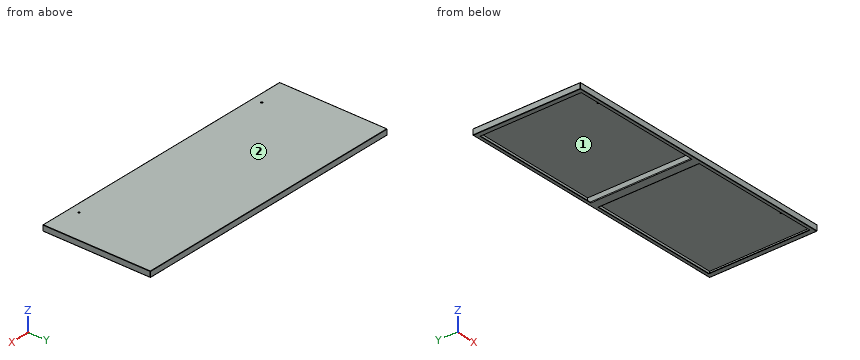
```python
from build123d import *

# Parameters (mm, degrees)
SKETCH_1_W          = 878
SKETCH_1_H          = 338
EXTRUDE_1_DEPTH     = 1.5
SKETCH_2_W          = 878
SKETCH_2_H          = 338
SKETCH_2_W_2        = 875
SKETCH_2_H_2        = 335
EXTRUDE_2_DEPTH     = 15
SKETCH_3_W          = 878
SKETCH_3_H          = 338
SKETCH_3_W_2        = 848
SKETCH_3_H_2        = 318
EXTRUDE_3_DEPTH     = 1.5
SKETCH_6_R          = 3
CUT_EXTRUDE_1_DEPTH = 471.750464684
FILLET_1_R          = 1
EXTRUDE_5_REACH     = 550.249
FILLET_START        = -159
FILLET_2_DEPTH      = 318
FILLET_START_2      = 133.01507
FILLET_2_2_DEPTH    = 34.48493


with BuildPart() as part:
    # 草图1 → 凸台-拉伸1 (new body)
    with BuildSketch(Plane.XY):
        Rectangle(SKETCH_1_W, SKETCH_1_H)
    extrude(amount=EXTRUDE_1_DEPTH)

    # 草图2 → 凸台-拉伸2 (add)
    with BuildSketch(Plane(origin=(0, 0, 0), x_dir=(-1, 0, 0), z_dir=(0, 0, -1))):
        Rectangle(SKETCH_2_W, SKETCH_2_H)
        Rectangle(SKETCH_2_W_2, SKETCH_2_H_2, mode=Mode.SUBTRACT)
    extrude(amount=EXTRUDE_2_DEPTH)

    # 草图3 → 凸台-拉伸3 (add)
    with BuildSketch(Plane(origin=(0, 0, -15), x_dir=(-1, 0, 0), z_dir=(0, 0, -1))):
        Rectangle(SKETCH_3_W, SKETCH_3_H)
        Rectangle(SKETCH_3_W_2, SKETCH_3_H_2, mode=Mode.SUBTRACT)
    extrude(amount=EXTRUDE_3_DEPTH)

    # 草图6 → 切除-拉伸1 (cut, through all)
    with BuildSketch(Plane.XY.offset(1.5)):
        with Locations((-339, -140)):
            Circle(SKETCH_6_R)
        with Locations((339, -140)):
            Circle(SKETCH_6_R)
    extrude(amount=-CUT_EXTRUDE_1_DEPTH, mode=Mode.SUBTRACT)

    # 圆角1
    fillet_1_edges = [part.edges().sort_by_distance(p)[0] for p in [
        (439, 0, 1.5),
        (0, 169, 1.5),
        (-439, 0, -16.5),
        (0, 169, -16.5),
        (439, 0, -16.5),
        (0, -169, -16.5),
        (-439, 0, 1.5),
        (0, -169, 1.5),
        (-439, 169, -7.5),
        (439, 169, -7.5),
        (439, -169, -7.5),
        (-439, -169, -7.5),
    ]]
    fillet(fillet_1_edges, radius=FILLET_1_R)

    # 草图9 → 凸台-拉伸5 (add, up to next)
    with BuildSketch(Plane(origin=(0, -159, 0), x_dir=(1, 0, 0), z_dir=(0, 1, 0)), mode=Mode.PRIVATE) as extrude_5_sk1:
        Polygon((15, 0), (15, 16.5), (-15, 16.5), (-15, 0), (-13.5, 0), (-13.5, 15), (13.5, 15), (13.5, 0), align=None)
    extrude_5_tool1 = extrude(extrude_5_sk1.sketch, amount=EXTRUDE_5_REACH, mode=Mode.PRIVATE) - part.part
    add(extrude_5_tool1.solids().sort_by_distance((14.657619, -159, -8.25))[0])

    # 圆角2: read off the stored shape, not the designer's step
    # 圆角2 outline → 圆角2 (cut)
    with BuildSketch(Plane(origin=(0, 0, 0), x_dir=(1, 0, 0), z_dir=(0, 1, 0)).offset(FILLET_START)):
        with BuildLine():
            ThreePointArc((-15, 14.5), (-14.414213562, 15.914213562), (-13, 16.5))
            Line((-13, 16.5), (-15, 16.5))
            Line((-15, 16.5), (-15, 14.5))
        make_face()
        with BuildLine():
            Line((15, 14.5), (15, 16.5))
            Line((15, 16.5), (13, 16.5))
            ThreePointArc((13, 16.5), (14.414213562, 15.914213562), (15, 14.5))
        make_face()
    extrude(amount=FILLET_2_DEPTH, mode=Mode.SUBTRACT)

    # Fillet 2 2 outline → Fillet 2 2 (cut)
    with BuildSketch(Plane(origin=(0, 0, 0), x_dir=(1, 0, 0), z_dir=(0, 1, 0)).offset(FILLET_START_2)):
        with BuildLine():
            Line((-15, 15), (-15, 14.5))
            ThreePointArc((-15, 14.5), (-14.984059392, 14.752008585), (-14.936491673, 15))
            Line((-14.936491673, 15), (-15, 15))
        make_face()
        with BuildLine():
            Line((15, 15), (14.936491673, 15))
            ThreePointArc((14.936491673, 15), (14.984059392, 14.752008585), (15, 14.5))
            Line((15, 14.5), (15, 15))
        make_face()
    extrude(amount=FILLET_2_2_DEPTH, mode=Mode.SUBTRACT)


solid = part.part
```
Could you check a few things on this model? Use its own coordinates, in mm. Face numbers are marked on the shaded views. Coordinates: 2 decimals unless noted, no trailing zeros. Loops run counter-clockwise (first coordinate to the right, second up) from the corner with the lowest first, then second, coordinate; pieces in that order, holes last. Notation, with made-up numbers: M 29.5,3.25 L 46.5,3.25 A13 ccw 46.5,22.25 Z; hole C 59,29 d11. An arc over 180 degrees is marked long. Put each result on its own line as item: value. Start each with the question number.
(1) Suppose I cut it at C-C on x = -275. Please give me the cut outline in (y, z).
(2) Thinking about a two-plate mould opening in Y: for the marked faces 1 and 2, which applies, pulls with the +Y half, pulls with the -Y half, needs draft (parallel to the pull), parting line crosses it, or undercut?
(3) Suppose I cut it at B-B on y = 142. Please give me the cut outline in (x, z), then the cut area to 3 significant figures.
(4) I need wall thicknesses on line 1 (X direction, y = 95.5, z = -13.5); line 2 (X direction, y = -140, z = 0.55); line 3 (Z direction, x = -3, y = -80). Which ranges of each line are inside material? Lowest first, please. Write a range as from..to.
(5) Will these pins go through, and if not, where does the flat tip stop? P1, Ø3, axis at x = 26, y = -19, coming from the -Z side; P2, Ø3.5, axis at x = 339, y = -140, coming from the +Z side.
(6) Suppose I cut it at A-A on z = -10. Please give me the cut outline in (x, y), then the cut area to 3 significant figures.
Solutions:
1. outline: M -169,-15.5 A1 ccw -168,-16.5 L -159,-16.5 L -159,-15 L -167.5,-15 L -167.5,0 L 167.5,0 L 167.5,-15 L 159,-15 L 159,-16.5 L 168,-16.5 A1 ccw 169,-15.5 L 169,0.5 A1 ccw 168,1.5 L -168,1.5 A1 ccw -169,0.5 Z
2. face 1: undercut
2. face 2: needs draft
3. outline: M -439,-15.5 A1 ccw -438,-16.5 L -424,-16.5 L -424,-15 L -437.5,-15 L -437.5,0 L -15,0 L -15,-14.5 A2 ccw -13,-16.5 L 13,-16.5 A2 ccw 15,-14.5 L 15,0 L 437.5,0 L 437.5,-15 L 424,-15 L 424,-16.5 L 438,-16.5 A1 ccw 439,-15.5 L 439,0.5 A1 ccw 438,1.5 L -438,1.5 A1 ccw -439,0.5 Z; hole M -13.5,-15 L 13.5,-15 L 13.5,0 L -13.5,0 Z
3. area: 1,490 mm2
4. line 1: x = -439..-437.5, -15..-13.5, 13.5..15, 437.5..439
4. line 2: x = -439..-342, -336..336, 342..439
4. line 3: z = -16.5..-15, 0..1.5
5. P1: stops at z = 0
5. P2: passes through
6. outline: M -439,-168 A1 ccw -438,-169 L 438,-169 A1 ccw 439,-168 L 439,168 A1 ccw 438,169 L -438,169 A1 ccw -439,168 Z; hole M -437.5,-167.5 L 437.5,-167.5 L 437.5,167.5 L 15,167.5 L 15,-159 L 13.5,-159 L 13.5,167.5 L -13.5,167.5 L -13.5,-159 L -15,-159 L -15,167.5 L -437.5,167.5 Z
6. area: 4,620 mm2
